Print and shaded views of the part. All mm, measured from the part's lowest x, y and z. Round coordinates to 2 decimals unless told otherwise and drop trailing zeros. Write each loop counter-clockwise with the first axis right and the second up, starting at its lowest first coordinate (ties: lowest second). Pieces come first, ordered by that corner, then holes. Notation, with made-up numbers: (50, 47) - (96, 47) arc R18 ccw to (96, 71) - close; hole circle Ø2 at (78.25, 60). An arc over 180 degrees is marked (long way). Answer as a JSON object with one key per item and string values. Group by question number.
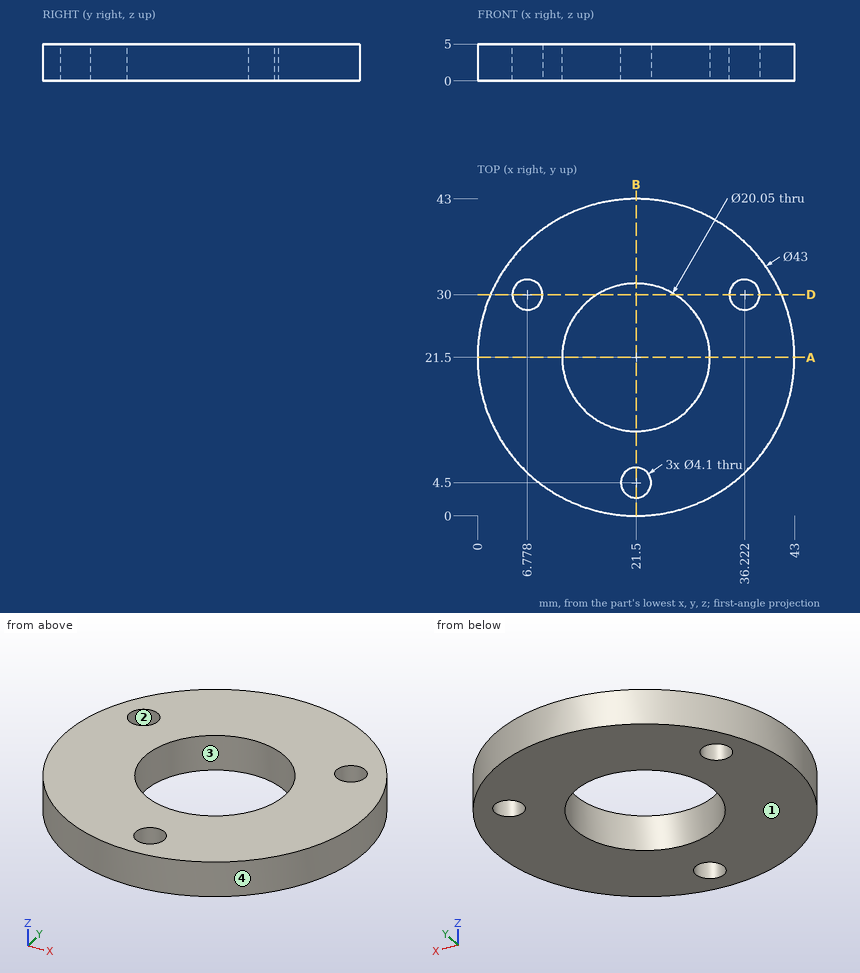
(1) Slice it at D-D (y = 30). Write the cut outline in (x, z) (1 decimal), then the cut area to 3 significant figures.
(2) Drill centre lines: line 1 (X direction, y = 29.5, z = 1.65) (1 decimal); line 2 (X direction, y = 5.5, z = 4.4); line 3 (Y direction, x = 15.5, z = 1.4) (1 decimal). Where is each one in solid material? Low to high. Write a range as from..to.
(3) Slice it at A-A (y = 21.5). Write the cut outline in (x, z) (1 decimal), then the cut area to 3 significant figures.
(4) Flat gauge pins, fed straight in: pin 1 (18 mm diameter, centred on x = 21.5, y = 21.5, fed in from +Z); pin 2 (2 mm diameter, centred on x = 28, z = 4.5, fed in from -Y) (1 decimal); pin 3 (1 mm diameter, centred on x = 18, z = 2.5, fed in from -Y); pin 4 (2 mm diameter, centred on x = 25.5, z = 3.5, fed in from +Y). Where does each tip first touch, or does it go through?
(5) Pull direction X, two halves, no side cores. Call the marked faces 1, 2, 3 and 4: pulls with the +X half, pulls with the -X half, needs draft (parallel to the pull), parting line crosses it, or undercut.
(6) Slice it at B-B (x = 21.5). Count the separate pieces of the cut face and the enclosed holes in it.
Answer:
{
 "1": {"outline": "(1.8, 0) - (4.7, 0) - (4.7, 5) - (1.8, 5) - close; (8.8, 0) - (16.2, 0) - (16.2, 5) - (8.8, 5) - close; (26.8, 0) - (34.2, 0) - (34.2, 5) - (26.8, 5) - close; (38.3, 0) - (41.2, 0) - (41.2, 5) - (38.3, 5) - close", "area": "103 mm²"},
 "2": {"line 1": "1.5..4.8, 8.8..15.5, 27.5..34.2, 38.2..41.5", "line 2": "7.14..19.71, 23.29..35.86", "line 3": "0.9..13.5, 29.5..42.1"},
 "3": {"outline": "(0, 0) - (11.5, 0) - (11.5, 5) - (0, 5) - close; (31.5, 0) - (43, 0) - (43, 5) - (31.5, 5) - close", "area": "115 mm²"},
 "4": {"pin 1": "through", "pin 2": "y = 0.7", "pin 3": "y = 0.21", "pin 4": "y = 42.79"},
 "5": {"face 1": "needs draft", "face 2": "undercut", "face 3": "undercut", "face 4": "parting line crosses it"},
 "6": {"separate pieces": "3", "enclosed holes": "0"}
}
